```python
from build123d import *

# Parameters (mm, degrees)
EXTRUDE_1_DEPTH     = 5
SKETCH_2_R          = 1.45
CUT_EXTRUDE_1_DEPTH = 5
CUT_EXTRUDE_2_DEPTH = 4
FILLET_1_R          = 10


with BuildPart() as part:
    # Эскиз1 → Бобышка-Вытянуть1 (new body)
    with BuildSketch(Plane(origin=(0, 0, 0), x_dir=(1, 0, 0), z_dir=(0, 1, 0))):
        with BuildLine():
            Line((25.256912811, 27.718916921), (27.395437576, 35.7))
            ThreePointArc((27.395437576, 35.7), (45, 0), (27.395437576, -35.7))
            Line((27.395437576, -35.7), (25.256912811, -27.718916921))
            ThreePointArc((25.256912811, -27.718916921), (37.5, 0), (25.256912811, 27.718916921))
        make_face()
    extrude(amount=EXTRUDE_1_DEPTH)

    # Эскиз2 → Вырез-Вытянуть1 (cut)
    with BuildSketch(Plane(origin=(0, 5, 0), x_dir=(1, 0, 0), z_dir=(0, 1, 0))):
        with Locations(Location((42.5, 0, 0), (0, 0, 270))):
            Circle(SKETCH_2_R)
        with Locations(Location((28.793836633, 31.259638065, 0), (0, 0, 270))):
            Circle(SKETCH_2_R)
        with Locations(Location((28.793836633, -31.259638065, 0), (0, 0, 90))):
            Circle(SKETCH_2_R)
    extrude(amount=-CUT_EXTRUDE_1_DEPTH, mode=Mode.SUBTRACT)

    # Эскиз3 → Вырез-Вытянуть2 (cut)
    with BuildSketch(Plane(origin=(0, 5, 0), x_dir=(1, 0, 0), z_dir=(0, 1, 0))):
        with BuildLine():
            Line((29.152397919, 28.734107513), (30.952735107, 29.657502375))
            ThreePointArc((30.952735107, 29.657502375), (40.5, -1.12e-07), (30.952736281, -29.657502977))
            Line((30.952736281, -29.657502977), (29.152399104, -28.734108121))
            ThreePointArc((29.152399104, -28.734108121), (38.5, -1.11e-07), (29.152397919, 28.734107513))
        make_face()
    extrude(amount=-CUT_EXTRUDE_2_DEPTH, mode=Mode.SUBTRACT)

    # Скругление1
    fillet_1_edges = [part.edges().sort_by_distance(p)[0] for p in [
        (25.256912811, 2.5, 27.718916921),
        (25.256912811, 2.5, -27.718916921),
    ]]
    fillet(fillet_1_edges, radius=FILLET_1_R)


solid = part.part
```
Work out the finished part from the listing and answer in its coordinate system (mm). A direction names the side the tool comes from. Give positions to 0.01 mm unless a question says otherwise; leave off trailing zeros. Loops run counter-clockwise (first coordinate to the right, second up) from the corner with the lowest first, then second, coordinate; pieces in that order, holes last. Notation, with made-up numbers: (62.5, -24.5) -> (97.5, -24.5) arc R31 ccw to (97.5, -0.5) -> close; hole circle Ø8 at (14, 47.5). An arc over 180 degrees is marked (long way). One line per question, with ' | ' between items. Start each with the question number.
1) Determine the mould class of faces 3 (the face through (26.593, 2.535, -28.452)), 4 (the face through (38, 5, 2)), 5 (the face through (40.5, 3, -0.4)) for opening direction X: +X half, -X half, draft (parallel to the pull), parting line (faces both ways), or undercut.
2) Section A-A, the plane z = 0 is taken. Determine the outline of the cut face in (x, y), then the cut area to 3 significant figures.
3) Section B-B, the plane x = 36 is taken. Determine the outline of the cut face in (y, z), then the cut area to 3 significant figures.
4) Section D-D, the plane z = 12.5 is taken. Determine the outline of the cut face in (x, y).
5) Each of these flat-tipped pins is pushed along its axis until it touches: pin 1 (1 mm diameter, centred on y = 3.5, z = 20, fed in from +X); pin 2 (1 mm diameter, centred on y = 3.5, z = -9.5, fed in from -X); pin 3 (2.5 mm diameter, centred on x = 28.79, z = -31.26, fed in from +Y); pin 4 (1 mm diameter, centred on x = 38.5, y = 3.5, fed in from +Z). Where does it stop, or does it pass through?
6) Section C-C, the plane y = 3.5 is taken. Determine the outline of the cut face in (x, z).
7) Straight lines are drawn through the part: L1, parallel to Z at x = 28.75, y = 4.3; L2, parallel to Z at x = 27.5, y = 2.4; L3, parallel to Z at x = 29.25, y = 4.8. For each, find the intervals that lie inside material, in ascending order.
8) For faces 1 (the face through (30.04, 3.03, -29.19)), 2 (the face through (27.57, 2.54, 30.48)), determine the directions among +Z, -Z, +X, -X, +Y, -Y from which every point of the face is accessible in a straight line to the end or side of a thin tool.
Resolved:
1) face 3: -X half | face 4: draft | face 5: undercut
2) outline: (37.5, 0) -> (41.05, 0) -> (41.05, 5) -> (40.5, 5) -> (40.5, 1) -> (38.5, 1) -> (38.5, 5) -> (37.5, 5) -> close; (43.95, 0) -> (45, 0) -> (45, 5) -> (43.95, 5) -> close | area: 15.0 mm2
3) outline: (0, -27) -> (5, -27) -> (5, -20.91) -> (1, -20.91) -> (1, -15.43) -> (5, -15.43) -> (5, -10.5) -> (0, -10.5) -> close; (0, 10.5) -> (5, 10.5) -> (5, 15.43) -> (1, 15.43) -> (1, 20.91) -> (5, 20.91) -> (5, 27) -> (0, 27) -> close | area: 121 mm2
4) outline: (35.36, 0) -> (43.23, 0) -> (43.23, 5) -> (38.94, 5) -> (38.94, 1) -> (36.87, 1) -> (36.87, 5) -> (35.36, 5) -> close
5) pin 1: x = 40.56 | pin 2: x = 36.14 | pin 3: through | pin 4: z = 24.1
6) outline: (26.71, -33.14) -> (27.4, -35.7) arc R45 ccw to (27.4, 35.7) -> (26.71, 33.14) arc R10 ccw to (28.71, 24.12) arc R37.5 cw to (28.71, -24.12) arc R10 ccw to start; hole circle Ø2.9 at (28.79, -31.26); hole circle Ø2.9 at (28.79, 31.26); hole (29.15, -28.73) -> (30.95, -29.66) arc R50.84 ccw to (30.95, 29.66) -> (29.15, 28.73) arc R48.84 cw to start; hole circle Ø2.9 at (42.5, 0)
7) L1: -34.62 to -32.71, -29.81 to -24.08, 24.08 to 29.81, 32.71 to 34.62 | L2: -35.62 to -31.91, -30.61 to -25.93, 25.93 to 30.61, 31.91 to 35.62 | L3: -34.2 to -32.64, -29.88 to -28.78, -28.6 to -23.47, 23.47 to 28.6, 28.78 to 29.88, 32.64 to 34.2
8) face 1: +Y | face 2: +Y, -Y
